The drawing under review shows one solid part. Ordinate dimensions are in mm from its lowest x, y, z. A direction names the side the tool comes from. Round coordinates to 2 decimals unless told otherwise and drop trailing zeros. Order: outer loops, then holes, each group sorted by start corner. A loop starts at its lowest first (then second) coordinate and runs counter-clockwise, first axis right, second up.
1) Consider section D-D (x = 81). Give the boundary of the cut face in (y, z) (1 decimal).
2) Mouldability with a two-part tool opening along X and no side actions: class the marked faces 3, 4 and 5 as pulls with the +X half, pulls with the -X half, needs draft (parallel to the pull), parting line crosses it, or undercut.
3) To check wall thickness, follow L1, parallel to Y at x = 82, z = 26 (1 decimal); L2, parallel to X at y = 90.5, z = 20 (1 decimal); L3, parallel to Z at x = 68, y = 21 (1 decimal). State the ranges of each line that lie inside material, in increasing order.
4) Consider section B-B (z = 18). Give the boundary of the cut face in (x, y) (1 decimal).
5) Clearance check with a flat-ended pin moving along its axis: P1, Ø12, axis at x = 54.5, y = 14.5, coming from the +Z side (1 decimal). State where the tip first meets the part, or that it passes through.
6) Consider section A-A (x = 29.5). Give the boundary of the cut face in (y, z) (1 decimal).
7) Machinability: for the marked faces 1 and 2, which of the approach directions +Z, -Z, +X, -X, +Y, -Y give a long, thin tool a straight path to every point of the face, cutting with its end or side? Answer none if there is none.
8) Consider section C-C (y = 109). Give the boundary of the cut face in (x, z) (1 decimal).
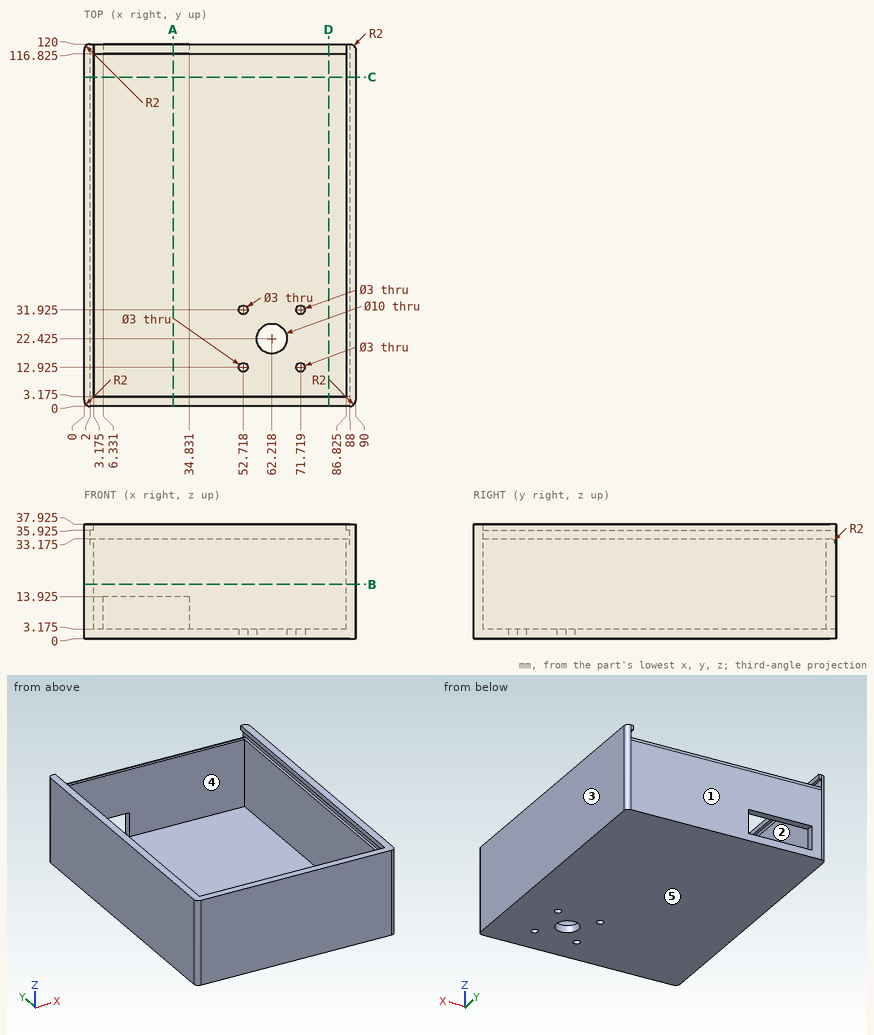
Answer below:
1. outline: (0, 0) - (120, 0) - (120, 31.2) arc R2 ccw to (118, 33.2) - (116.8, 33.2) - (116.8, 3.2) - (3.2, 3.2) - (3.2, 37.9) - (0, 37.9) - close
2. face 3: pulls with the +X half
2. face 4: undercut
2. face 5: needs draft
3. L1: y = 0 to 3.2, 116.8 to 120
3. L2: x = 0 to 3.2, 86.8 to 90
3. L3: z = 0 to 3.2
4. outline: (0, 2) arc R2 ccw to (2, 0) - (88, 0) arc R2 ccw to (90, 2) - (90, 118) arc R2 ccw to (88, 120) - (2, 120) arc R2 ccw to (0, 118) - close; hole (3.2, 3.2) - (86.8, 3.2) - (86.8, 116.8) - (3.2, 116.8) - close
5. P1: stops at z = 3.2
6. outline: (0, 0) - (120, 0) - (120, 3.2) - (3.2, 3.2) - (3.2, 37.9) - (0, 37.9) - close; (116.8, 13.9) - (120, 13.9) - (120, 31.2) arc R2 ccw to (118, 33.2) - (116.8, 33.2) - close
7. face 1: +Z, -Z, +X, -X, +Y
7. face 2: +Z
8. outline: (0, 0) - (90, 0) - (90, 37.9) - (86.8, 37.9) - (86.8, 35.9) - (88, 35.9) - (88, 33.2) - (86.8, 33.2) - (86.8, 3.2) - (3.2, 3.2) - (3.2, 33.2) - (2, 33.2) - (2, 35.9) - (3.2, 35.9) - (3.2, 37.9) - (0, 37.9) - close
